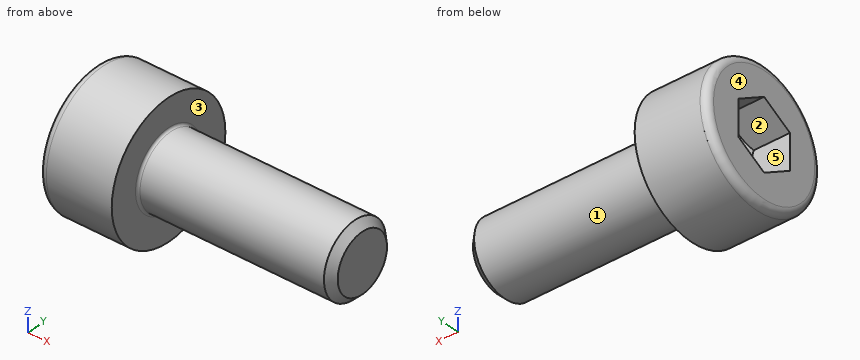
Autodesk Inventor part; units mm, degrees
ref_plane "Work Plane1" through (30, 0, 0) normal (0, -0.5, 0.866) x (1, 0, 0)
ref_plane "YZ Plane" through (0, 0, 0) normal (1, 0, 0) x (0, 1, 0)
ref_plane "XZ Plane" through (0, 0, 0) normal (0, 1, 0) x (-1, 0, 0)
sketch "Sketch1" plane through (0, 0, 0) normal (0, 0, 1) x (1, 0, 0)
  line L0 (-0.6667, 0) -> (8, 0)
  line L1 (8, 0) -> (8, 1.5)
  line L2 (8, 1.5) -> (1.3067, 1.5)
  line L3 (1.3067, 1.5) -> (1, 1.5)
  line L4 (1, 1.5) -> (0, 1.5)
  line L5 (0, 1.5) -> (0, 2.75)
  line L6 (0, 2.75) -> (-3, 2.75)
  line L7 (-3, 2.75) -> (-3, 1.4434)
  line L8 (-3, 1.4434) -> (-1.5, 1.4434)
  line L9 (-1.5, 1.4434) -> (-0.6667, 0)
  line L10 (-5.2, 0) -> (10.2, 0)
  line L11 (0, -0.55) -> (0, 3.3)
  line L12 (1.3067, 1.5) -> (0, 1.5) construction
  dimension "d0" = 6.6933
  dimension "d1" = 0.3067
  dimension "d2" = 3
  dimension "d3" = 1.5
  dimension "d4" = 60
  dimension "d5" = 3
  dimension "d6" = 3
  dimension "d7" = 2.8868
  dimension "d8" = 5.5
  dimension "d19" = 8
revolve "Body" add sketch "Sketch1" angle 360 about axis through (-0.6667, 0, 0) along (1, 0, 0)
sketch "Sketch2" plane through (-3, 0, 0) normal (-1, 0, 0) x (0, 0, 1)
  circle A0 centre (0, 0) radius 1.4434
  line L0 (0, -3.85) -> (0, 3.85)
  line L1 (-3.85, 0) -> (3.85, 0)
  line L2 (1.4434, 0) -> (0.7217, -1.25)
  line L3 (0.7217, -1.25) -> (-0.7217, -1.25)
  line L4 (-0.7217, -1.25) -> (-1.4434, 0)
  line L5 (-1.4434, 0) -> (-0.7217, 1.25)
  line L6 (-0.7217, 1.25) -> (0.7217, 1.25)
  line L7 (0.7217, 1.25) -> (1.4434, 0)
extrude "Slot" add sketch "Sketch2" against normal up to next contours L7 A0 | A0 L2 | L6 L0 A0 | A0 L0 L3 | L0 L6 A0 | A0 L3 L0 | L4 A0 | A0 L5
fillet "Fillet2" radius 0.3 1 edges at (-3, -2.75, 0)
thread "Thread"
chamfer "Chamfer1" distance 0.3067 distance2 0.3067 1 edges at (8, -1.5, 0) measured on face at (8, 0.5539, 0.4443)
fillet "Fillet1" radius 0.1 1 edges at (0, -1.5, 0)
ref_plane "Work Plane1" through (30, 0, 0) normal (0, -0.5, 0.866) x (1, 0, 0)
equation "\"d0\" = GEL"
equation "\"d1\" = GAL"
equation "\"d2\" = KOH"
equation "\"d3\" = INTI"
equation "\"d5\" = GD"
equation "\"d6\" = BDM"
equation "\"d7\" = 1.1547 * SW"
equation "\"d8\" = KOD"
equation "\"d19\" = NLG"
equation "\"d16\" = RR"
equation "\"d12\" = GEL"
equation "\"d14\" = -0.5 * SPD + 0.5 * GD"
equation "\"d15\" = GUL"
equation "\"d29\" = R"
equation "\"GD\" = NND"
equation "\"NLG\" = 8"
equation "\"GEL\" = 6.69328"
equation "\"KOD\" = 5.5"
equation "\"KOH\" = 3"
equation "\"INTI\" = 1.5"
equation "\"GAL\" = 0.61345 * PTC"
equation "\"GUL\" = 0.61345 * PTC"
equation "\"BDM\" = NND"
equation "\"SW\" = 2.5"
equation "\"RR\" = 0.3"
equation "\"SPD\" = 2.38655"
equation "\"d28\" = R"
equation "\"R\" = 0.1"
equation "\"TOA\" = 30deg"
equation "\"THREADDIA\" = 3"
equation "\"KOD1\" = KOD"
equation "\"PTC\" = 0.5"
equation "\"NND\" = 3"
equation "\"E0\" = 1.155 * SW"
equation "\"GD1\" = THREADDIA - 1.2269 * PTC"
properties part number "ANSI B18.3.1M - M3x0.5 x 8, BSHCSM" material "Steel, Mild"
Design review of the part built by this model. Coordinates are the model's own, in mm. Face numbers are marked on the shaded views. A direction names the side the tool comes from. Coordinates: 2 decimals unless noted, no trailing zeros. Order: outer loops, then holes, each group sorted by start corner. A loop starts at its lowest first (then second) coordinate and runs counter-clockwise, first axis right, second up.
1) For the marked faces 4 and 5, list the 3-axis set-ups (+Z, -Z, +X, -X, +Y, -Y) from which the entire face can be reached by the end or side of a thin tool; tool diameter is ignored.
2) Clearance check with flat-ended pins moving along their axes: pin 1 (0.7 mm diameter, centred on x = -2, z = -0.5, fed in from +Y); pin 2 (1.2 mm diameter, centred on x = -2.5, z = 0.5, fed in from -Y). State where each tip first meets the part, or that it passes through.
3) Wall thickness on line 1 along X through (y, z) = (2.1, 1.2); line 2 along Z through (x, y) = (0.5, 0.4); line 3 along Y through (x, z) = (-2, -1.1): over which ranges is each line inside the solid? List them lowest first.
4) Take a section at A-A, the plane x = -0.5. Give the boundary of the cut face in (y, z), and give its area (3 significant figures).
5) Take a section at B-B, the plane x = 1. Give the boundary of the cut face in (y, z), and give its area (3 significant figures).
6) Mouldability with a two-part tool opening along Y and no side actions: class the marked faces 1, 2 and 3 as +Y half, -Y half, draft (parallel to the pull), parting line (faces both ways), or undercut.
Returned:
1. face 4: +Z, -Z, -X, +Y, -Y
1. face 5: -X
2. pin 1: stops at y = 2.75
2. pin 2: stops at y = -2.75
3. line 1: x = -3 to 0
3. line 2: z = -1.45 to 1.45
3. line 3: y = -2.52 to -0.59, 0.59 to 2.52
4. outline: circle Ø5.5 at (0, 0)
4. area: 23.8 mm2
5. outline: circle Ø3 at (0, 0)
5. area: 7.07 mm2
6. face 1: parting line
6. face 2: undercut
6. face 3: draft
